from build123d import *

# Parameters (mm, degrees)
F0_W         = 95.3711643815
F0_H         = 77.4655118585
F1_DEPTH     = 10.16
F2_T         = -6.35
F3_DEPTH     = 5.588
F4_DEPTH     = 3.8735
F5_DEPTH     = 0.5715
F6_DEPTH     = 7.62
F7_W         = 83.6853682995
F7_H         = 57.4865713716
F7_H_2       = 9.9894702435
F8_DEPTH     = 58.9915
F9_DEPTH     = 5.715
F10_T4_DEPTH = 413.7319634586


# Not quite as in the source:
# - a fillet or chamfer that OpenCascade refuses, or shapes differently, is made with other operations: its cross-section is extruded or revolved along the edge and cut away or added


with BuildPart() as f1:
    # F0 (on Front) → F1 (new body)
    with BuildSketch(Plane.XZ):
        Rectangle(F0_W, F0_H)
    extrude(amount=-F1_DEPTH)

    # F2
    f2_openings = [f1.faces().sort_by_distance(p)[0] for p in [
        (0, 0, 0),
    ]]
    offset(amount=F2_T, openings=f2_openings)

    # F3 (add): a face of the model
    f3_faces = [f1.faces().sort_by_distance(p)[0] for p in [
        (0, 3.81, 0),
    ]]
    extrude(f3_faces, amount=F3_DEPTH)

    # F4 (cut): a face of the model
    f4_faces = [f1.faces().sort_by_distance(p)[0] for p in [
        (0, -1.778, 0),
    ]]
    extrude(f4_faces, amount=-F4_DEPTH, mode=Mode.SUBTRACT)

    # F5 (cut): a face of the model
    f5_faces = [f1.faces().sort_by_distance(p)[0] for p in [
        (0, 2.0955, 0),
    ]]
    extrude(f5_faces, amount=-F5_DEPTH, mode=Mode.SUBTRACT)

    # F6 (add): a face of the model
    f6_faces = [f1.faces().sort_by_distance(p)[0] for p in [
        (0, 10.16, 0),
    ]]
    extrude(f6_faces, amount=F6_DEPTH)

    # F7 (on face) → F8 (join)
    with BuildSketch(Plane(origin=(0, 17.78, 0), x_dir=(-1, 0, 0), z_dir=(0, 1, 0))):
        Rectangle(F7_W, F7_H)
        with Locations((0, -33.7380208075)):
            Rectangle(F7_W, F7_H_2)
    extrude(amount=F8_DEPTH)

    # F9 (add): a face of the model
    f9_faces = [f1.faces().sort_by_distance(p)[0] for p in [
        (0, 47.27575, 28.7432856858),
    ]]
    extrude(f9_faces, amount=F9_DEPTH)

    # F10: chamfer of 63.5 x 10.16 on 1 edges, made by hand


with BuildPart() as f10_tool2:
    # F10_s3 → F10_t4 (new body)
    with BuildSketch(Plane.YZ.offset(-206.8659817293)):
        Polygon((13.2715, 34.4582856858), (76.7715, 24.2982856858), (76.7715, 34.4582856858), align=None)
    extrude(amount=F10_T4_DEPTH)

    split(bisect_by=Plane.XZ.offset(-17.78), keep=Keep.BOTTOM)


with BuildPart() as f1_1:
    add(f1.part)

    # F10_t1: cut F10_tool2
    add(f10_tool2.part, mode=Mode.SUBTRACT)


solid = f1_1.part
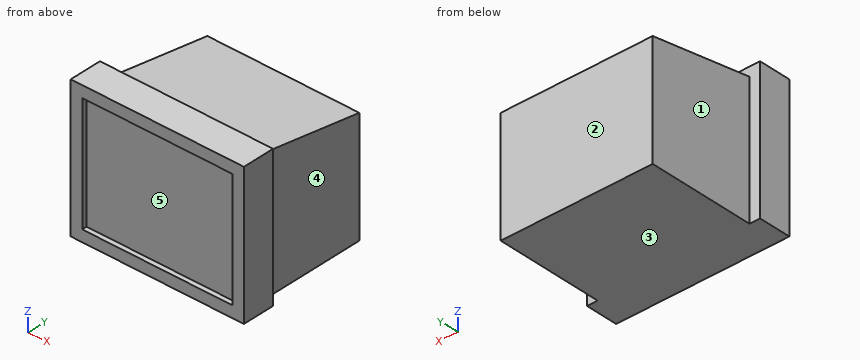
The listing builds one solid part. Answer for the finished solid, in the listing's coordinates (mm). Face numbers are marked on the shaded views. A direction names the side the tool comes from. Give positions to 0.01 mm unless a question says otherwise; leave off trailing zeros. Loops run counter-clockwise (first coordinate to the right, second up) from the corner with the lowest first, then second, coordinate; pieces in that order, holes last. Notation, with made-up numbers: (87, 78.25) - (145, 78.25) arc R8 ccw to (145, 82.25) - close; hole circle Ø7 at (-14.5, 35). An arc over 180 degrees is marked (long way). Answer as a JSON object with one key per item and string values.
1. Find the intervals of material crossed by L1, parallel to X at y = 73, z = -3.5; L2, parallel to Y at x = 42, z = -29.5; L3, parallel to Y at x = 11.5, z = -1, in increasing order. Write a range as [from, to].
Determined:
{"L1": "[-41.84, 41.84]", "L2": "[0, 17.78]", "L3": "[2.67, 76.77]"}
2. For a pull along Z with two mould halves and no side action, classify the marked faces 3, 4 and 5 as pulls with the +Z half, pulls with the -Z half, needs draft (parallel to the pull), parting line crosses it, or undercut.
Determined:
{"face 3": "pulls with the -Z half", "face 4": "needs draft", "face 5": "undercut"}
3. For the marked faces 1 and 2, determine the directions among +Z, -Z, +X, -X, +Y, -Y from which every point of the face is accessible in a straight line to the end or side of a thin tool.
Determined:
{"face 1": "+Z, -Z, -X, +Y", "face 2": "+Z, -Z, +X, -X, +Y"}
4. A cutting plane is placed at C-C (y = 39). Write down the section's boundary in (x, z), then the cut area to 3 significant figures.
Determined:
{"outline": "(-41.84, -38.73) - (41.84, -38.73) - (41.84, 30.34) - (-41.84, 30.34) - close", "area": "5,780 mm²"}
5. Flat-ended cylindrical pins translate along their axes: pin 1 Ø1 at (x, z) = (-27.5, -11) entering from -Y; pin 2 Ø1.5 at (y, z) = (35.5, 8.5) entering from -X; pin 3 Ø1 at (x, y) = (6, 25.5) entering from +Z. Find the tip coordinate at first contact, or state that the pin passes through.
Determined:
{"pin 1": "y = 2.67", "pin 2": "x = -41.84", "pin 3": "z = 32.58"}
6. A cutting plane is placed at A-A (x = 9.5). Write down the section's boundary in (y, z), then the cut area to 3 significant figures.
Determined:
{"outline": "(0, -38.73) - (76.77, -38.73) - (76.77, 24.3) - (17.78, 33.74) - (17.78, 38.73) - (0, 38.73) - (0, 32.38) - (2.67, 32.38) - (2.67, -32.38) - (0, -32.38) - close", "area": "5,200 mm²"}
7. A cutting plane is placed at D-D (y = 29). Write down the section's boundary in (x, z).
Determined:
{"outline": "(-41.84, -38.73) - (41.84, -38.73) - (41.84, 31.94) - (-41.84, 31.94) - close"}
8. A cutting plane is placed at B-B (z = -28). Write down the section's boundary in (x, y).
Determined:
{"outline": "(-47.69, 0) - (-41.34, 0) - (-41.34, 2.67) - (41.34, 2.67) - (41.34, 0) - (47.69, 0) - (47.69, 17.78) - (41.84, 17.78) - (41.84, 76.77) - (-41.84, 76.77) - (-41.84, 17.78) - (-47.69, 17.78) - close"}
